Autodesk Inventor part; units mm, degrees
ref_plane "YZ Plane" through (0, 0, 0) normal (1, 0, 0) x (0, 1, 0)
ref_plane "XZ Plane" through (0, 0, 0) normal (0, 1, 0) x (-1, 0, 0)
ref_plane "XY Plane" through (0, 0, 0) normal (0, 0, 1) x (1, 0, 0)
sketch "main" plane through (0, 0, 0) normal (0, 0, 1) x (1, 0, 0)
  circle A0 centre (-191.7635, 49.9495) radius 2.1844
  circle A1 centre (-95.8324, -13.8772) radius 2.1
  arc A2 (-99.5462, -18.9735) -> (-92.0695, -8.7075) centre (-95.8064, -13.8415) ccw
  arc A3 (-198.1111, 49.7757) -> (-191.7635, 43.5995) centre (-191.7635, 49.9495) ccw
  line L0 (-200.5697, 139.5363) -> (-198.1111, 49.7757)
  arc A4 (-199.0195, 139.7975) -> (-92.0695, -8.7075) centre (80.274, 228.1743) ccw
  circle A5 centre (-195.1368, 115.1254) radius 2.0828
  line L1 (-191.7635, 43.5995) -> (-186.2072, 43.5995)
  arc A6 (-199.0195, 139.7975) -> (-200.5697, 139.5363) centre (-199.7762, 139.5581) ccw
  circle A7 centre (-135.2274, 18.1995) radius 2.0828
  circle A8 centre (-191.7635, 8.6745) radius 2.1844
  arc A9 (-191.7635, 15.0245) -> (-193.2141, 2.4924) centre (-191.7635, 8.6745) ccw
  line L2 (-185.4135, 15.8183) -> (-185.4135, 42.8058)
  line L3 (-191.7635, 15.0245) -> (-186.2072, 15.0245)
  arc A10 (-185.4135, 42.8058) -> (-186.2072, 43.5995) centre (-186.2072, 42.8058) ccw
  arc A11 (-186.2072, 15.0245) -> (-185.4135, 15.8183) centre (-186.2072, 15.8183) ccw
  line L4 (-193.2141, 2.4924) -> (-97.2571, -20.0236)
  point P0 (1.1251, 9.7944)
  point P1 (-200.7302, 145.398)
  dimension "d7" = 12.7
  dimension "d8" = 4.1656
  dimension "d9" = 6.35
  dimension "d11" = 0.7937
  dimension "d13" = 4.1656
  dimension "d15" = 12.7
  dimension "d16" = 0.7937
sketch "Sketch1" plane through (0, 0, 0) normal (1, 0, 0) x (0, 1, 0)
  circle A0 centre (0, 0) radius 2.1844
  circle A1 centre (95.9311, -63.8268) radius 2.1
  arc A2 (92.2173, -68.923) -> (99.694, -58.6571) centre (95.9571, -63.7911) ccw
  arc A3 (-6.3476, -0.1739) -> (0, -6.35) centre (0, 0) ccw
  line L0 (-8.8062, 89.5868) -> (-6.3476, -0.1739)
  arc A4 (-7.256, 89.848) -> (99.694, -58.6571) centre (272.0375, 178.2247) ccw
  circle A5 centre (-3.3733, 65.1759) radius 2.0828
  line L1 (0, -6.35) -> (5.5563, -6.35)
  arc A6 (-7.256, 89.848) -> (-8.8062, 89.5868) centre (-8.0127, 89.6085) ccw
  circle A7 centre (56.5361, -31.75) radius 2.0828
  circle A8 centre (0, -41.275) radius 2.1844
  arc A9 (0, -34.925) -> (-1.4506, -47.4571) centre (0, -41.275) ccw
  line L2 (6.35, -34.1313) -> (6.35, -7.1438)
  line L3 (0, -34.925) -> (5.5563, -34.925)
  arc A10 (6.35, -7.1438) -> (5.5563, -6.35) centre (5.5563, -7.1437) ccw
  arc A11 (5.5563, -34.925) -> (6.35, -34.1313) centre (5.5563, -34.1313) ccw
  line L4 (-1.4506, -47.4571) -> (94.5064, -69.9732)
extrude "Extrusion1" add sketch "Sketch1" along normal blind 1.5875
properties part number "ramp"
Source: CAD feature listing. Evaluate the final solid. Frame: model axes, mm. A direction names the side the tool comes from. Coordinates: 2 decimals unless noted, no trailing zeros. Loops run counter-clockwise (first coordinate to the right, second up) from the corner with the lowest first, then second, coordinate; pieces in that order, holes last. Notation, with made-up numbers: M 52.5,5 L 99.5,5 A21 cw 99.5,30 Z; hole C 68.5,59.5 d6. An arc over 180 degrees is marked long. Use a Markdown table: item, result. Add a question column.
Q1. Section query B-B, the plane z = -31.75. Return loops of the section in (x, y).
Q2. Section query A-A, the plane x = 0.4. State how many separate pieces and enclosed holes the cut face has, and give its area (3 significant figures).
Q3. Material intervals for L1, parallel to Y at x = 1, z = 1.5; L2, parallel to Y at x = 0.85, z = -17; L3, parallel to Y at x = 1.55, z = 43, sorted ascending.
Q4. Section query D-D, the plane z = 25.5. Return loops of the section in (x, y).
Q5. First-contact query: pin 1 (4 mm diameter, centred on y = 0, z = 0, fed in from -X); pin 2 (7 mm diameter, centred on y = 0, z = -41.275, fed in from +X); pin 3 (0.8 mm diameter, centred on x = 1, y = 3.5, fed in from +Z). Flat tips, straight axial feed; report the tip coordinate or a pass-through.
Q6. Access query for faces 1 (the cylindrical face through (0.78, -4.38, -4.6)), 2 (the cylindrical face through (0.78, 35.09, 5.97)). Directions: +Z, -Z, +X, -X, +Y, -Y. A direction counts if a zero-diameter tool reaches every point of the face in a straight line with its end or side. Return the directions, or none.
Q7. Section query C-C, the plane y = 33.5. Return loops of the section in (x, z).
Q8. Draft query along Z for faces 3 (the cylindrical face through (0.783, 101.779, -66.326)), 4 (the cylindrical face through (0.78, -3.82, 67.21)), 5 (the flat face through (1.588, 30, -13)). Return one class per face: pulls with the +Z half, pulls with the -Z half, needs draft (parallel to the pull), parting line crosses it, or undercut.
Result:
| question | item | result |
|---|---|---|
| 1 | outline | M 0,6.35 L 1.59,6.35 L 1.59,54.45 L 0,54.45 Z; M 0,58.62 L 1.59,58.62 L 1.59,67.77 L 0,67.77 Z |
| 2 | separate pieces | 1 |
| 2 | enclosed holes | 5 |
| 2 | area | 5,690 mm2 |
| 3 | L1 | y = -6.39 to -1.59, 1.59 to 38.41 |
| 3 | L2 | y = 6.35 to 53.63 |
| 3 | L3 | y = -7.53 to 12.17 |
| 4 | outline | M 0,-7.05 L 1.59,-7.05 L 1.59,22.06 L 0,22.06 Z |
| 5 | pin 1 | passes through |
| 5 | pin 2 | stops at x = 1.59 |
| 5 | pin 3 | stops at z = 62.09 |
| 6 | face 1 | +X, -X, -Y |
| 6 | face 2 | +Z, +X, -X, +Y |
| 7 | outline | M 0,-55.66 L 1.59,-55.66 L 1.59,8.18 L 0,8.18 Z |
| 8 | face 3 | parting line crosses it |
| 8 | face 4 | undercut |
| 8 | face 5 | needs draft |
